```python
from build123d import *

# Parameters (mm, degrees)
F1_DEPTH = 63.5
F0_W     = 25.4
F0_H     = 19.05
F2_DEPTH = 25.4
F3_DEPTH = 7.9375
F5_R     = 6.35


with BuildPart() as f1:
    # F0 (on Front) → F1 (new body, symmetric)
    with BuildSketch(Plane.XZ):
        Polygon((22.225, 9.525), (-41.275, 9.525), (-41.275, -9.525), (41.275, -9.525), (41.275, 9.525), align=None)
    extrude(amount=F1_DEPTH, both=True)

    # F0 (on Front) → F2 (join, symmetric)
    with BuildSketch(Plane.XZ):
        with Locations((73.025, 52.4002)):
            Rectangle(F0_W, F0_H)
        with BuildLine():
            Line((22.225, 27.0002), (22.225, 9.525))
            Line((22.225, 9.525), (41.275, 9.525))
            Line((41.275, 9.525), (41.275, 27.0002))
            ThreePointArc((41.275, 27.0002), (45.9246798487, 38.2255201513), (57.15, 42.8752))
            Line((57.15, 42.8752), (60.325, 42.8752))
            Line((60.325, 42.8752), (60.325, 61.9252))
            Line((60.325, 61.9252), (57.15, 61.9252))
            add(Edge.make_bspline(
                [(56.6424278756, 61.9215114808), (56.8121178687, 61.9231320915), (56.981311275, 61.924361744), (57.15, 61.9252)],
                knots=[110.9960891503, 110.9960891503, 110.9960891503, 110.9960891503, 111.5045361635, 111.5045361635, 111.5045361635, 111.5045361635], degree=3))
            ThreePointArc((56.6424278756, 61.9215114808), (32.275489136, 51.5157936962), (22.225, 27.0002))
        make_face()
    extrude(amount=F2_DEPTH, both=True)

    # F0 (on Front) → F3 (join, symmetric)
    with BuildSketch(Plane.XZ):
        with BuildLine():
            add(Edge.make_bspline(
                [(-41.275, 9.525), (-41.1113175395, 42.5821639465), (19.5983994664, 61.5677254569), (56.6424278756, 61.9215114808)],
                knots=[0, 0, 0, 0, 110.9960891503, 110.9960891503, 110.9960891503, 110.9960891503], degree=3))
            Line((-41.275, 9.525), (22.225, 9.525))
            Line((22.225, 9.525), (22.225, 27.0002))
            ThreePointArc((22.225, 27.0002), (32.275489136, 51.5157936962), (56.6424278756, 61.9215114808))
        make_face()
    extrude(amount=F3_DEPTH, both=True)

    # F0 (on Front) → F4 (revolve)
    with BuildSketch(Plane.XZ):
        Polygon((85.725, 66.675), (85.725, 61.9252), (85.725, 42.8752), (85.725, 38.1), (111.125, 38.1), (111.125, 66.675), align=None)
    revolve(axis=Axis((85.725, 0, 52.3875), (0, 0, 1)))

    # F5
    f5_edges = [f1.edges().sort_by_distance(p)[0] for p in [
        (41.275, -63.5, 0),
        (-41.275, -63.5, 0),
        (41.275, 63.5, 0),
        (-41.275, 63.5, 0),
    ]]
    fillet(f5_edges, radius=F5_R)


solid = f1.part
```
Here's how the part is built. I have some questions about the finished solid (model axes, mm). A direction names the side the tool comes from. Give positions to 0.01 mm unless a question says otherwise; leave off trailing zeros. Order: outer loops, then holes, each group sorted by start corner. A loop starts at its lowest first (then second) coordinate and runs counter-clockwise, first axis right, second up. Notation, with made-up numbers: (6, 45) -> (48, 45) arc R12 cw to (48, 66) -> close; hole circle Ø9 at (36.25, 83). An arc over 180 degrees is marked (long way). Use CSV: the item, a comma, the result in double quotes. Start each with the question number.
Item 1: I'm going to push flat-ended pins straight in: P1, Ø15, axis at x = 82.5, y = 9, coming from the -Z side; P2, Ø8.5, axis at y = -19, z = 19.5, coming from the -X side (3 decimals); P3, Ø16.5, axis at x = -19, y = 35.5, coming from the +Z side (3 decimals). Where does each tip first touch, or does it pass through?
Item 2: On a 3-axis mill with a long thin cutter (end or side, diameter ignored), from which of +Z, -Z, +X, -X, +Y, -Y can I reach the whole of each face in a straight line? I mean faces 1 (the flat face through (41.275, -1, 4)), 2 (the cylindrical face through (45.8, -0.4, 38.1)), 3 (the flat face through (-3, 7.938, 30)). Say none if no direction works.
Item 3: Suppose I cut it at A-A (y = -33.5). List the corners of the cut face in (x, z) for me (3 decimals).
Item 4: If I drill on probe 1 along Z at (x, y) = (3.5, -53.5) (3 decimals); probe 2 along Y at (x, z) = (8, 25); probe 3 along Z at (x, y) = (57, -16), over which ranges is the centre line in solid material (lowest first)? Write a range as [from, to].
Answer block:
1,P1,"stops at z = 38.1"
1,P2,"stops at x = 22.225"
1,P3,"stops at z = 9.525"
2,face 1,"-Z, +X, +Y, -Y"
2,face 2,"-Z, +Y, -Y"
2,face 3,"+Z, -X, +Y"
3,outline,"(-41.275, -9.525) -> (41.275, -9.525) -> (41.275, 9.525) -> (-41.275, 9.525) -> close"
4,probe 1,"z = [-9.525, 9.525]"
4,probe 2,"y = [-7.94, 7.94]"
4,probe 3,"z = [42.87, 61.92]"
